Read the model definition and answer for the solid it produces. Units are mm, in the model's axes. Give positions to 0.01 mm unless a question says otherwise; leave off trailing zeros. Loops run counter-clockwise (first coordinate to the right, second up) from the corner with the lowest first, then second, coordinate; pieces in that order, holes last. Notation, with made-up numbers: (44.25, 12.5) -> (49.25, 12.5) arc R21 ccw to (49.25, 22.5) -> close; hole circle Ø5 at (-14.75, 52). An arc over 180 degrees is marked (long way). Write each question's results on one line, items separated by ' | '. Start each with the question number.
Item 1: Section B-B on y = 8.25 is taken. State how many separate pieces and enclosed holes the cut face has, and give its area (3 significant figures).
Item 2: Section A-A on x = 38 is taken. Write down the section's boundary in (y, z), and give its area (3 significant figures).
Item 3: Find the intervals of material crossed by line 1 (Y direction, x = -38, z = 32); line 2 (Z direction, x = -36, y = 9.5); line 3 (Z direction, x = -5.5, y = 8), in increasing order.
Item 4: Each of these flat-tipped pins is pushed along its axis until it touches: P1, Ø4, axis at y = 4, z = 1, coming from the +X side; P2, Ø4, axis at y = 2, z = 15.5, coming from the -X side; P3, Ø1.5, axis at y = 3.5, z = -2.5, coming from the +X side. Where does it stop, or does it pass through?
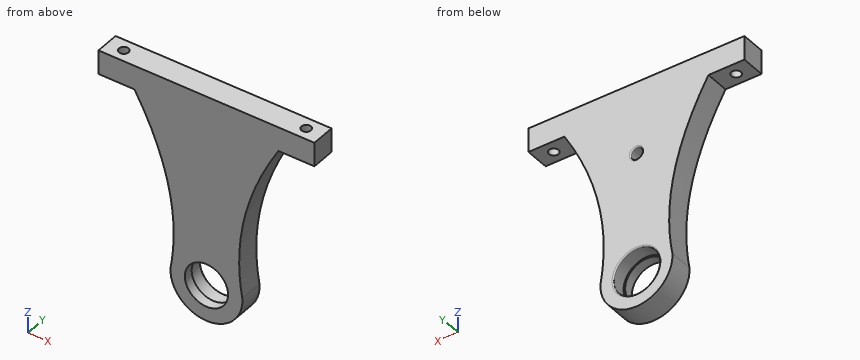
```python
from build123d import *

# Parameters (mm, degrees)
EXTRUDE_1_DEPTH     = 10
SKETCH_2_R          = 9.65
CUT_EXTRUDE_1_DEPTH = 6
SKETCH_3_R          = 9
CUT_EXTRUDE_2_DEPTH = 5.0000001
SKETCH_4_R          = 2
CUT_EXTRUDE_3_DEPTH = 11.0000001
SKETCH_5_R          = 2.5
CUT_EXTRUDE_4_DEPTH = 8
FILLET_1_R          = 0.5
FILLET_2_R          = 0.5


with BuildPart() as part:
    # Эскиз1 → Бобышка-Вытянуть1 (new body)
    with BuildSketch(Plane(origin=(0, 0, 0), x_dir=(1, 0, 0), z_dir=(0, 1, 0))):
        with BuildLine():
            Line((-45, -37.036390428), (45, -37.036390428))
            Line((45, -37.036390428), (45, -27.036390428))
            Line((45, -27.036390428), (30, -27.036390428))
            add(Edge.make_bspline(
                [(30, -27.036390428), (8.982189831, 8.482679734), (14.96841635, 41.990721102)],
                knots=[0, 0, 0, 0.673052388, 0.673052388, 0.673052388], degree=2))
            ThreePointArc((14.96841635, 41.990721102), (0, 57.963609572), (-14.96841635, 41.990721102))
            add(Edge.make_bspline(
                [(-30, -27.036390428), (-8.982189831, 8.482679734), (-14.96841635, 41.990721102)],
                knots=[0, 0, 0, 0.673052388, 0.673052388, 0.673052388], degree=2))
            Line((-30, -27.036390428), (-45, -27.036390428))
            Line((-45, -27.036390428), (-45, -37.036390428))
        make_face()
    extrude(amount=EXTRUDE_1_DEPTH)

    # Эскиз2 → Вырез-Вытянуть1 (cut)
    with BuildSketch(Plane(origin=(0, 10, 0), x_dir=(1, 0, 0), z_dir=(0, 1, 0))):
        with Locations((0, 42.963609572)):
            Circle(SKETCH_2_R)
    extrude(amount=-CUT_EXTRUDE_1_DEPTH, mode=Mode.SUBTRACT)

    # Эскиз3 → Вырез-Вытянуть2 (cut, through all)
    with BuildSketch(Plane(origin=(0, 4, 0), x_dir=(1, 0, 0), z_dir=(0, 1, 0))):
        with Locations((0, 42.963609572)):
            Circle(SKETCH_3_R)
    extrude(amount=-CUT_EXTRUDE_2_DEPTH, mode=Mode.SUBTRACT)

    # Эскиз4 → Вырез-Вытянуть3 (cut, through all)
    with BuildSketch(Plane(origin=(0, 0, 27.036390428), x_dir=(-1, 0, 0), z_dir=(0, 0, -1))):
        with Locations((38, 5)):
            Circle(SKETCH_4_R)
        with Locations((-38, 5)):
            Circle(SKETCH_4_R)
    extrude(amount=-CUT_EXTRUDE_3_DEPTH, mode=Mode.SUBTRACT)

    # Эскиз5 → Вырез-Вытянуть4 (cut)
    with BuildSketch(Plane(origin=(0, 10, 0), x_dir=(1, 0, 0), z_dir=(0, 1, 0))):
        with Locations((0, -7.036390428)):
            Circle(SKETCH_5_R)
    extrude(amount=-CUT_EXTRUDE_4_DEPTH, mode=Mode.SUBTRACT)

    # Скругление1
    fillet_1_edges = [part.edges().sort_by_distance(p)[0] for p in [
        (-2.5, 10, 7.036390428),
    ]]
    fillet(fillet_1_edges, radius=FILLET_1_R)

    # Скругление2
    fillet_2_edges = [part.edges().sort_by_distance(p)[0] for p in [
        (-9.65, 10, -42.963609572),
    ]]
    fillet(fillet_2_edges, radius=FILLET_2_R)


solid = part.part
```
Findings:
1) separate pieces: 1 | enclosed holes: 2 | area: 3,460 mm2
2) outline: (0, 27.04) -> (3, 27.04) -> (3, 37.04) -> (0, 37.04) -> close; (7, 27.04) -> (10, 27.04) -> (10, 37.04) -> (7, 37.04) -> close | area: 60.0 mm2
3) line 1: 0 to 3, 7 to 10 | line 2: 27.04 to 37.04 | line 3: -56.92 to -50.89, -35.03 to 37.04
4) P1: x = 18.79 | P2: x = -24.83 | P3: x = 17.31
